Design review of the part built by this model. Coordinates are the model's own, in mm. Give positions to 0.01 mm unless a question says otherwise; leave off trailing zeros. Loops run counter-clockwise (first coordinate to the right, second up) from the corner with the lowest first, then second, coordinate; pieces in that order, holes last. Notation, with made-up numbers: (72.25, 20) -> (97.25, 20) arc R12 cw to (97.25, 31) -> close; hole circle Ø4 at (-27.5, -18.75). An arc over 180 degrees is marked (long way). Answer as CSV lines item,"result".
from build123d import *

# Parameters (mm, degrees)
F0_W     = 12.7
F0_H     = 12.7
F1_DEPTH = 12.7
F2_R     = 2.54
F3_DEPTH = 25.4
F4_R     = 2.54
F5_DEPTH = 25.4
F6_R     = 2.54
F7_DEPTH = 25.4


with BuildPart() as f1:
    # F0 (on Top) → F1 (new body)
    with BuildSketch(Plane.XY):
        Rectangle(F0_W, F0_H)
    extrude(amount=F1_DEPTH)

    # F2 (on face) → F3 (cut)
    with BuildSketch(Plane(origin=(-6.35, 0, 0), x_dir=(0, -1, 0), z_dir=(-1, 0, 0))):
        with Locations((0, 6.35)):
            Circle(F2_R)
    extrude(amount=-F3_DEPTH, mode=Mode.SUBTRACT)

    # F4 (on face) → F5 (cut)
    with BuildSketch(Plane.XZ.offset(6.35)):
        with Locations((0, 6.35)):
            Circle(F4_R)
    extrude(amount=-F5_DEPTH, mode=Mode.SUBTRACT)

    # F6 (on face) → F7 (cut)
    with BuildSketch(Plane.XY.offset(12.7)):
        Circle(F6_R)
    extrude(amount=-F7_DEPTH, mode=Mode.SUBTRACT)


solid = f1.part
Q1. The part is to be moulded in two halves that separate along Z. For faces 1 (the flat face through (3, 0, 0)), 2 (the flat face through (3, 0, 12.7)), 3 (the cylindrical face through (-4.105, 2.538, 6.462)), 4 (the flat face through (3, -6.35, 6)), say which applies: pulls with the +Z half, pulls with the -Z half, needs draft (parallel to the pull), parting line crosses it, or undercut.
Filled sheet:
face 1,"pulls with the -Z half"
face 2,"pulls with the +Z half"
face 3,"undercut"
face 4,"needs draft"
Q2. To check wall thickness, follow probe 1 along Z at (x, y) = (0, -4.9); probe 2 along Y at (x, z) = (0, 10.85); probe 3 along Y at (x, z) = (-2, 10.25). State the ranges of each line that lie inside material, in increasing order. Write a range as from..to.
Filled sheet:
probe 1,"z = 0..3.81, 8.89..12.7"
probe 2,"y = -6.35..-2.54, 2.54..6.35"
probe 3,"y = -6.35..-1.57, 1.57..6.35"
Q3. Clearance check with a flat-ended pin moving along its axis: pin 1 Ø4 at (x, y) = (0, 0) entering from +Z (3 decimals). State where the tip first meets the part, or that it passes through.
Filled sheet:
pin 1,"passes through"
Q4. We need section A-A, the plane y = 0. State the section outline as (x, z) points.
Filled sheet:
outline,"(-6.35, 0) -> (-2.54, 0) -> (-2.54, 3.81) -> (-6.35, 3.81) -> close; (-6.35, 8.89) -> (-2.54, 8.89) -> (-2.54, 12.7) -> (-6.35, 12.7) -> close; (2.54, 0) -> (6.35, 0) -> (6.35, 3.81) -> (2.54, 3.81) -> close; (2.54, 8.89) -> (6.35, 8.89) -> (6.35, 12.7) -> (2.54, 12.7) -> close"
Q5. We need section C-C, the plane y = -4.5. State the section outline as (x, z) points.
Filled sheet:
outline,"(-6.35, 0) -> (6.35, 0) -> (6.35, 12.7) -> (-6.35, 12.7) -> close; hole circle Ø5.08 at (0, 6.35)"
Q6. We need section D-D, the plane z = 9.5. State the section outline as (x, y) points, and give its area (3 significant figures).
Filled sheet:
outline,"(-6.35, -6.35) -> (6.35, -6.35) -> (6.35, 6.35) -> (-6.35, 6.35) -> close; hole circle Ø5.08 at (0, 0)"
area,"141 mm^2"
